Geometry: final body of the model. Coordinates: model frame, mm. Face numbers are marked on the shaded views. A direction names the side the tool comes from. Give positions to 0.01 mm unless a question says otherwise; leave off trailing zeros. Loops run counter-clockwise (first coordinate to the right, second up) from the corner with the lowest first, then second, coordinate; pieces in that order, holes last. Notation, with made-up numbers: (6, -33.75) -> (15, -33.75) arc R18 cw to (15, -12.75) -> close; hole circle Ø6 at (80.25, 1). An arc over 180 degrees is marked (long way). Answer in a Markdown table with one row per item. Add a question column.
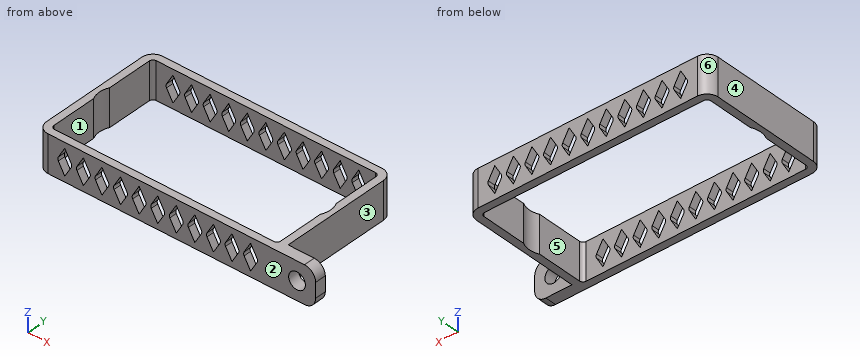
from build123d import *

# Parameters (mm, degrees)
BOSS_EXTRUDE1_DEPTH = 5
SKETCH2_R           = 2.25
CUT_EXTRUDE1_DEPTH  = 54.735463151
FILLET1_R           = 3
CUT_EXTRUDE2_DEPTH  = 56.601258979
LPATTERN1_COUNT     = 6
LPATTERN1_PITCH     = 5
LPATTERN1_COL_COUNT = 6
LPATTERN1_COL_PITCH = 5


with BuildPart() as part:
    # Sketch1 → Boss-Extrude1 (new, symmetric)
    with BuildSketch(Plane.XY):
        with BuildLine():
            Line((-32.5, -14.75), (-32.5, 14.75))
            ThreePointArc((-32.5, 14.75), (-31.621320344, 16.871320344), (-29.5, 17.75))
            Line((-29.5, 17.75), (29.5, 17.75))
            ThreePointArc((29.5, 17.75), (31.621320344, 16.871320344), (32.5, 14.75))
            Line((32.5, 14.75), (32.5, -14.75))
            Line((32.5, -14.75), (42.5, -14.75))
            Line((42.5, -14.75), (42.5, -17.75))
            Line((42.5, -17.75), (29.5, -17.75))
            Line((29.5, -17.75), (-29.5, -17.75))
            ThreePointArc((-29.5, -17.75), (-31.621320344, -16.871320344), (-32.5, -14.75))
        make_face()
        with BuildLine():
            Line((-29.5, -15.75), (29.5, -15.75))
            ThreePointArc((29.5, -15.75), (30.207106781, -15.457106781), (30.5, -14.75))
            Line((30.5, -14.75), (30.5, -2.5))
            ThreePointArc((30.5, -2.5), (31.090169944, 0), (30.5, 2.5))
            Line((30.5, 2.5), (30.5, 14.75))
            ThreePointArc((30.5, 14.75), (30.207106781, 15.457106781), (29.5, 15.75))
            Line((29.5, 15.75), (-29.5, 15.75))
            ThreePointArc((-29.5, 15.75), (-30.207106781, 15.457106781), (-30.5, 14.75))
            Line((-30.5, 14.75), (-30.5, 2.5))
            ThreePointArc((-30.5, 2.5), (-31.090169944, 0), (-30.5, -2.5))
            Line((-30.5, -2.5), (-30.5, -14.75))
            ThreePointArc((-30.5, -14.75), (-30.207106781, -15.457106781), (-29.5, -15.75))
        make_face(mode=Mode.SUBTRACT)
    extrude(amount=BOSS_EXTRUDE1_DEPTH, both=True)

    # Sketch2 → Cut-Extrude1 (cut, through all)
    with BuildSketch(Plane(origin=(0, -14.75, 0), x_dir=(1, 0, 0), z_dir=(0, 1, 0))):
        with Locations(Location((37.5, 0, 0), (0, 0, 180))):
            Circle(SKETCH2_R)
    extrude(amount=-CUT_EXTRUDE1_DEPTH, mode=Mode.SUBTRACT)

    # Fillet1
    fillet1_edges = [part.edges().sort_by_distance(p)[0] for p in [
        (42.5, -16.25, -5),
        (42.5, -16.25, 5),
    ]]
    fillet(fillet1_edges, radius=FILLET1_R)

    # Sketch3 → Cut-Extrude2 (cut, through all)
    with BuildSketch(Plane.XZ.offset(17.75)):
        with BuildLine():
            Line((0, -3.5), (1.732050808, -0.5))
            ThreePointArc((1.732050808, -0.5), (1.866025404, 0), (1.732050808, 0.5))
            Line((1.732050808, 0.5), (0, 3.5))
            Line((0, 3.5), (-1.732050808, 0.5))
            ThreePointArc((-1.732050808, 0.5), (-1.866025404, 0), (-1.732050808, -0.5))
            Line((-1.732050808, -0.5), (0, -3.5))
        make_face()
    cut_extrude2 = extrude(amount=-CUT_EXTRUDE2_DEPTH, mode=Mode.SUBTRACT)

    # LPattern1: Cut-Extrude2 ×6
    with Locations(*[(-i * LPATTERN1_PITCH, 0, 0) for i in range(1, LPATTERN1_COUNT)]):
        add(cut_extrude2, mode=Mode.SUBTRACT)

    # LPattern1 col: Cut-Extrude2 ×6
    with Locations(*[(i * LPATTERN1_COL_PITCH, 0, 0) for i in range(1, LPATTERN1_COL_COUNT)]):
        add(cut_extrude2, mode=Mode.SUBTRACT)


solid = part.part
(1) Draft query along Y for the marked faces 4, 5 and 6. Return one class per face: +Y half, -Y half, draft (parallel to the pull), parting line (faces both ways), or undercut.
(2) Cut plane A-A on x = 37.5. Return the cut outline in (y, z).
(3) Material intervals for line 1 along Z through (x, y) = (37.5, -15.75); line 2 along X through (y, z) = (0, -3.5); line 3 along Y through (x, z) = (2, -0.5), sorted ascending. Write a range as from..to.
(4) Reachability of the marked faces 1, 2 and 3 from +Z, -Z, +X, -X, +Y, -Y: full face, straight path, thin tool, end or side. Return the list, or none.
(5) Pin query (flat end, axial travel): pin 1 Ø5 at (x, z) = (36.5, 2.5) entering from +Y; pin 2 Ø2.5 at (x, z) = (37.5, 0) entering from -Y; pin 3 Ø3 at (y, z) = (-10, 0.5) entering from +X. Return the tip coordinate at first contact, or that it passes through.
(6) Cut plane B-B on y = -5. Return the cut outline in (x, z), then the cut area to 3 significant figures.
Answer list:
| question | item | result |
|---|---|---|
| 1 | face 4 | draft |
| 1 | face 5 | undercut |
| 1 | face 6 | +Y half |
| 2 | outline | (-17.75, -5) -> (-14.75, -5) -> (-14.75, -2.25) -> (-17.75, -2.25) -> close; (-17.75, 2.25) -> (-14.75, 2.25) -> (-14.75, 5) -> (-17.75, 5) -> close |
| 3 | line 1 | z = -5..-2.25, 2.25..5 |
| 3 | line 2 | x = -32.5..-31.09, 31.09..32.5 |
| 3 | line 3 | y = -17.75..-15.75, 15.75..17.75 |
| 4 | face 1 | +Z, -Z |
| 4 | face 2 | +Z, -Z, +X, -X, -Y |
| 4 | face 3 | +Z, -Z, +X, +Y |
| 5 | pin 1 | stops at y = -14.75 |
| 5 | pin 2 | passes through |
| 5 | pin 3 | stops at x = 32.5 |
| 6 | outline | (-32.5, -5) -> (-30.5, -5) -> (-30.5, 5) -> (-32.5, 5) -> close; (30.5, -5) -> (32.5, -5) -> (32.5, 5) -> (30.5, 5) -> close |
| 6 | area | 40.0 mm² |
